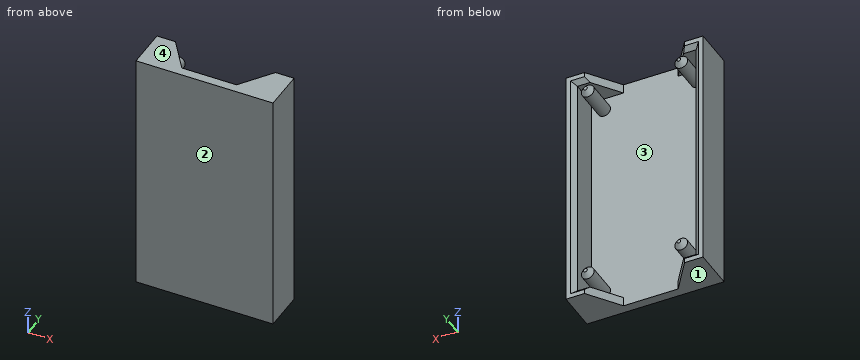
Autodesk Inventor part; units mm, degrees
ref_plane "YZ Plane" through (0, 0, 0) normal (1, 0, 0) x (0, 1, 0)
ref_plane "XZ Plane" through (0, 0, 0) normal (0, 1, 0) x (-1, 0, 0)
ref_plane "XY Plane" through (0, 0, 0) normal (0, 0, 1) x (1, 0, 0)
sketch "Sketch1" plane through (0, 0, 0) normal (0, 1, 0) x (-1, 0, 0)
  line L0 (0, 0) -> (26, 0)
  line L1 (26, 0) -> (26, -50)
  line L2 (26, -50) -> (0, -50)
  line L3 (0, -50) -> (0, 0)
  line L4 (28, 2) -> (-2, 2)
  line L5 (-2, 2) -> (-2, -52)
  line L6 (-2, -52) -> (28, -52)
  line L7 (28, -52) -> (28, 2)
  circle A0 centre (2.775, -2.78) radius 1.4
  circle A1 centre (23.225, -2.78) radius 1.4
  line L8 (2.775, -2.78) -> (23.225, -2.78) construction
  line L9 (26, -25) -> (0, -25) construction
  circle A2 centre (2.775, -47.22) radius 1.4
  circle A3 centre (23.225, -47.22) radius 1.4
  line L10 (2.775, -47.22) -> (23.225, -47.22) construction
  point P0 (13, 0)
  point P1 (13, -2.78)
  point P2 (13, -47.22)
  dimension "d0" = 2
  dimension "d1" = 50
  dimension "d2" = 26
  dimension "d3" = 2.8
  dimension "d4" = 2.8
  dimension "d5" = 23.25
  dimension "d6" = 0
  dimension "d7" = 1.38
extrude "Extrusion1" add sketch "Sketch1" against normal blind 2 contours L0 L1 L2 L3 | L7 L6 L5 L4 | A0 | A1 | A2 | A3
extrude "Extrusion2" add sketch "Sketch1" along normal blind 7 contours L7 L6 L5 L4
extrude "Extrusion3" add sketch "Sketch1" along normal blind 8 contours A0 | A1 | A2 | A3
chamfer "Chamfer1" distance 1 angle 45 8 edges at (-1.375, 8, -2.78) (-21.825, 8, -47.22) (-13, 7, -50) (-26, 7, -25) (0, 7, -25) (-1.375, 8, -47.22) (-21.825, 8, -2.78) (-13, 7, 0)
sketch "Sketch2" plane through (-28, -2, 2) normal (0, 0, 1) x (1, 0, 0)
  line L0 (29, 9) -> (1, 9)
  line L1 (28, 2) -> (28, 8)
  line L2 (2.0702, 9) -> (28, 9)
  line L3 (28, 9) -> (28, 2)
  line L4 (28, 2) -> (2.0702, 2)
  line L5 (2.0702, 2) -> (2.0702, 9)
  line L6 (25.9502, 9) -> (20.9781, 2)
  line L7 (0, 0) -> (30, 0)
  line L8 (15, 0) -> (15, 8)
  line L9 (4.0498, 9) -> (9.0219, 2)
extrude "Extrusion4" cut sketch "Sketch2" against normal blind 2 contours L6 L4 L9 L0
ref_plane "Work Plane1" through (-26, 0, -25) normal (0, 0, 1) x (1, 0, 0)
mirror "Mirror1" about plane through (-26, 0, -25) normal (0, 0, 1) of "Extrusion4"
properties part number "relay board holder"
Work out the finished part from the listing and answer in its coordinate system (mm). Face numbers are marked on the shaded views. Round coordinates to 2 decimals unless told otherwise and drop trailing zeros. Write each loop counter-clockwise with the first axis right and the second up, starting at its lowest first coordinate (ties: lowest second). Pieces come first, ordered by that corner, then holes.
1) Given pin 1 Ø1 at (x, z) = (-16, -28) entering from +Y; pin 2 Ø4.5 at (x, z) = (-25, -29.5) entering from +Y; pin 3 Ø1 at (x, y) = (-7, 2) entering from +Z; pin 4 Ø1.2 at (x, z) = (-0.5, -22) entering from +Y, each flat-ended and moving along its own axis, determine where each tip first touches the part or whether it passes through.
2) A cutting plane is placed at A-A (y = 4.5). Give the vertices of the cut face in (x, z) (3 decimals).
3) A cutting plane is placed at B-B (z = -9.5). Give the vertices of the cut face in (x, y).
4) A cutting plane is placed at C-C (x = -18). Give the vertices of the cut face in (y, z).
5) Straight lines are drawn through the part: line 1 (X direction, y = 5.5, z = -44.5); line 2 (Z direction, x = -22.25, y = 2); line 3 (Z direction, x = -25, y = 3.5). For each, find the intervals that lie inside material, in ascending order.
6) The mould has two halves that part along Z. Classify the marked faces 1, 2, 3 and 4: pulls with the +Z half, pulls with the -Z half, needs draft (parallel to the pull), parting line crosses it, or undercut.
Completed:
1. pin 1: stops at y = 0
1. pin 2: stops at y = 7
1. pin 3: passes through
1. pin 4: stops at y = 6.1
2. outline: (-28, -52) - (-22.174, -52) - (-22.174, -50) - (-26, -50) - (-26, 0) - (-22.174, 0) - (-22.174, 2) - (-28, 2) - close; circle Ø2.8 at (-23.225, -47.22); circle Ø2.8 at (-23.225, -2.78); circle Ø2.8 at (-2.775, -47.22); circle Ø2.8 at (-2.775, -2.78); (-3.826, -52) - (2, -52) - (2, 2) - (-3.826, 2) - (-3.826, 0) - (0, 0) - (0, -50) - (-3.826, -50) - close
3. outline: (-28, -2) - (2, -2) - (2, 7) - (1, 7) - (0, 6) - (0, 0) - (-26, 0) - (-26, 6) - (-27, 7) - (-28, 7) - close
4. outline: (-2, -52) - (0, -52) - (0, 2) - (-2, 2) - close
5. line 1: x = -28 to -26, 0 to 2
5. line 2: z = -52 to -50, -48.22 to -46.22, -3.78 to -1.78, 0 to 2
5. line 3: z = -52 to -50, 0 to 2
6. face 1: pulls with the -Z half
6. face 2: needs draft
6. face 3: undercut
6. face 4: pulls with the +Z half
